Answer from the drawing. Dimensions are ordinates in mm from the lowest x, y and z of the part. A direction names the side the tool comes from. Coordinates: 2 decimals unless noted, no trailing zeros. Order: outer loops, then holes, each group sorted by start corner. A loop starts at its lowest first (then second) coordinate and runs counter-clockwise, first axis right, second up. Notation, with made-up numbers: M 55.25,-37 L 62.25,-37 A24 cw 62.25,-26 Z; hole C 29,81 d11. An arc over 180 degrees is marked long. Use a Markdown table: item, result.
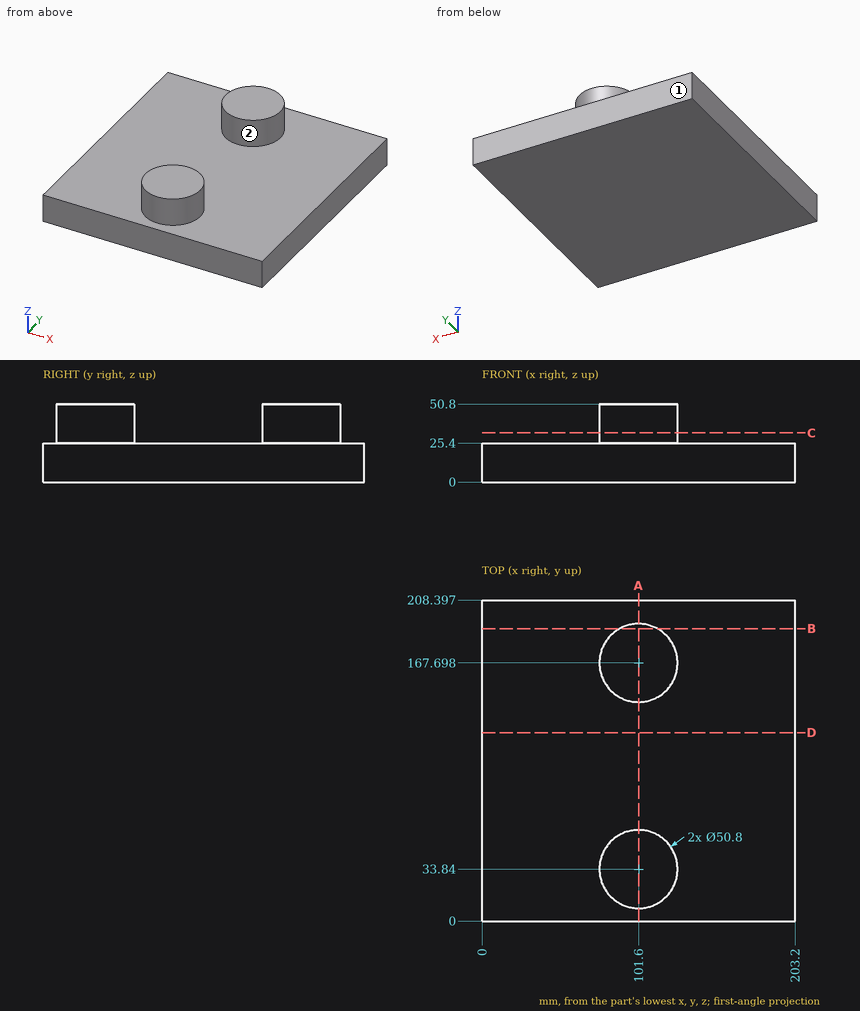
(1) A cutting plane is placed at C-C (z = 32). Determine the outline of the cut face in (x, y).
Conclusion:
| item | result |
|---|---|
| outline | C 101.6,33.84 d50.8; C 101.6,167.7 d50.8 |
(2) Straight lines are drawn through the part: L1, parallel to Z at x = 113.5, y = 95; L2, parallel to X at y = 53, z = 45.5 (1 decimal); L3, parallel to X at y = 29.5, z = 45. For each, find the intervals that lie inside material, in ascending order.
Conclusion:
| item | result |
|---|---|
| L1 | 0 to 25.4 |
| L2 | 84.9 to 118.3 |
| L3 | 76.57 to 126.63 |
(3) Given P1, Ø5, axis at x = 68.5, z = 29, coming from the +Y side; P2, Ø5, axis at x = 169.5, y = 81.5, coming from the -Z side; P3, Ø2, axis at x = 119.5, z = 32.5, coming from the +Y side; P4, Ø5, axis at y = 47, z = 41.5, coming from the +X side (1 decimal), each flat-ended and moving along its own axis, determine where each tip first touches the part or whether it passes through.
Conclusion:
| item | result |
|---|---|
| P1 | through |
| P2 | z = 0 |
| P3 | y = 186.66 |
| P4 | x = 124.7 |
(4) Which of the six approach directions +Z, -Z, +X, -X, +Y, -Y give full straight-line access (tool end or side, diameter ignored) to the marked faces 1 and 2?
Conclusion:
| item | result |
|---|---|
| face 1 | +Z, -Z, +X, -X, +Y |
| face 2 | +Z |
(5) A cutting plane is placed at D-D (y = 122.5). Determine the outline of the cut face in (x, z).
Conclusion:
| item | result |
|---|---|
| outline | M 0,0 L 203.2,0 L 203.2,25.4 L 0,25.4 Z |
(6) A cutting plane is placed at B-B (y = 190). Determine the outline of the cut face in (x, z), then the cut area to 3 significant figures.
Conclusion:
| item | result |
|---|---|
| outline | M 0,0 L 203.2,0 L 203.2,25.4 L 113.76,25.4 L 113.76,50.8 L 89.44,50.8 L 89.44,25.4 L 0,25.4 Z |
| area | 5,780 mm2 |
(7) A cutting plane is placed at A-A (x = 101.6). Determine the outline of the cut face in (y, z).
Conclusion:
| item | result |
|---|---|
| outline | M 0,0 L 208.4,0 L 208.4,25.4 L 193.1,25.4 L 193.1,50.8 L 142.3,50.8 L 142.3,25.4 L 59.24,25.4 L 59.24,50.8 L 8.44,50.8 L 8.44,25.4 L 0,25.4 Z |
